Model file for the job. Use its own axes, mm. Face numbers are marked on the shaded views. A direction names the side the tool comes from. Round coordinates to 2 decimals unless told otherwise and drop trailing zeros. Order: outer loops, then holes, each group sorted by start corner. A loop starts at its lowest first (then second) coordinate and runs counter-clockwise, first axis right, second up. Notation, with made-up numbers: M 26,25.25 L 49,25.25 A25 ccw 49,64.25 Z; hole C 40.25,46.5 d5. An arc over 180 degrees is marked long. Return JSON: item names as keys, results as strings. Group by question number.
Item 1: Slice it at D-D on y = 83.5. Write the cut outline in (x, z), then the cut area to 3 significant figures.
Item 2: Slice it at B-B on y = 7. Write the cut outline in (x, z).
Item 3: Slice it at C-C on z = -30. Write the cut outline in (x, y), then the cut area to 3 significant figures.
Item 4: Pin check, flat tips, straight feed: pin 1 Ø3.5 at (x, y) = (89.9, 80) entering from +Z; pin 2 Ø5.5 at (x, y) = (89.9, 80) entering from -Z; pin 3 Ø1.5 at (x, z) = (34, -49) entering from +Y; pin 4 Ø5.5 at (x, z) = (70, -45) entering from -Y. Stop position of each tip, or through.
Item 5: Which spindle directions (+Z, -Z, +X, -X, +Y, -Y) get a long thin tool onto all of the face, cutting with end or side? Do the marked faces 1 and 2. Say none if no direction does.
Item 6: Probe line 1 along Z through (x, y) = (70, 6.5); line 2 along X through (y, z) = (80, -56); line 3 along X through (y, z) = (23.5, -30). List the from-to ranges inside material, lowest first.
Item 7: Pull direction X, two halves, no side cores. Call the marked faces 3, 4, 5 and 6: pulls with the +X half, pulls with the -X half, needs draft (parallel to the pull), parting line crosses it, or undercut.
Item 8: Slice it at A-A on x = 25. Write the cut outline in (y, z), then the cut area to 3 significant figures.
from build123d import *

# Parameters (mm, degrees)
SKETCH1_W                  = 100
SKETCH1_H                  = 100
BOSS_EXTRUDE1_DEPTH        = 100
SKETCH2_W                  = 60
SKETCH2_H                  = 100
CUT_EXTRUDE1_DEPTH         = 174.205080757
CUT_EXTRUDE2_DEPTH         = 157.212427483
CUT_EXTRUDE2_DEPTH_BACK    = 157.212427483
SKETCH3_R                  = 11
SKETCH4_W                  = 40
SKETCH4_H                  = 100
CUT_EXTRUDE3_DEPTH         = 174.205080757
BOSS_EXTRUDE2_START        = -10.65
SKETCH5_R                  = 11
SKETCH5_R_2                = 8
BOSS_EXTRUDE2_DEPTH        = 10.65
M5_TAPPED_HOLE1_AT_2_COUNT = 2
M5_TAPPED_HOLE1_AT_2_PITCH = 60
M5_TAPPED_HOLE2_D          = 4.2
M5_TAPPED_HOLE2_DEPTH      = 22
M5_TAPPED_HOLE2_TIP        = 1.2618073
M8_TAPPED_HOLE1_D          = 6.8
M8_TAPPED_HOLE1_DEPTH      = 24.25
M8_TAPPED_HOLE1_TIP        = 2.042926105
FILLET3_R                  = 10


with BuildPart() as part:
    # Sketch1 → Boss-Extrude1 (new body)
    with BuildSketch(Plane(origin=(0, 0, 0), x_dir=(1, 0, 0), z_dir=(0, 1, 0))):
        with Locations((50, 50)):
            Rectangle(SKETCH1_W, SKETCH1_H)
    extrude(amount=BOSS_EXTRUDE1_DEPTH)

    # Sketch2 → Cut-Extrude1 (cut, through all)
    with BuildSketch(Plane.XY):
        with Locations((30, 83.65)):
            Rectangle(SKETCH2_W, SKETCH2_H)
    extrude(amount=-CUT_EXTRUDE1_DEPTH, mode=Mode.SUBTRACT)

    # Sketch3 → Cut-Extrude2 (cut, two sides: drawn at the far end of the back side and taken through both)
    with BuildSketch(Plane(origin=(0, 33.65, 0), x_dir=(1, 0, 0), z_dir=(0, 1, 0)).offset(-CUT_EXTRUDE2_DEPTH_BACK)):
        with Locations(Location((25, 30, 0), (0, 0, 270))):
            Circle(SKETCH3_R)
    extrude(amount=CUT_EXTRUDE2_DEPTH + CUT_EXTRUDE2_DEPTH_BACK, mode=Mode.SUBTRACT)

    # Sketch4 → Cut-Extrude3 (cut, through all)
    with BuildSketch(Plane.ZY):
        with Locations((-80, 50)):
            Rectangle(SKETCH4_W, SKETCH4_H)
    extrude(amount=-CUT_EXTRUDE3_DEPTH, mode=Mode.SUBTRACT)

    # Sketch5 → Boss-Extrude2 (add)
    with BuildSketch(Plane.XZ.offset(BOSS_EXTRUDE2_START)):
        with Locations(Location((25, -30, 0), (0, 0, 270))):
            Circle(SKETCH5_R)
        with Locations(Location((25, -30, 0), (0, 0, 270))):
            Circle(SKETCH5_R_2, mode=Mode.SUBTRACT)
    extrude(amount=BOSS_EXTRUDE2_DEPTH)

    # Sketch11 → M5 Tapped Hole1 (revolve, cut)
    with BuildSketch(Plane(origin=(89.9, 80, 0), x_dir=(0, -1, 0), z_dir=(1, 0, 0))):
        Polygon((0, 0), (0, 16.2618073), (2.1, 15), (2.1, 0), align=None)
    m5_tapped_hole1 = revolve(axis=Axis((89.9, 80, 6.35), (0, 0, -1)), mode=Mode.SUBTRACT)

    # M5 Tapped Hole1 at 2: M5 Tapped Hole1 ×2
    with Locations(*[(0, -i * M5_TAPPED_HOLE1_AT_2_PITCH, 0) for i in range(1, M5_TAPPED_HOLE1_AT_2_COUNT)]):
        add(m5_tapped_hole1, mode=Mode.SUBTRACT)

    # Mirror1: M5 Tapped Hole1 across plane
    add(m5_tapped_hole1.mirror(Plane.XY.offset(-30)), mode=Mode.SUBTRACT)

    # Mirror1 copy 1 sketch → Mirror1 copy 1 (revolve, cut)
    with BuildSketch(Plane(origin=(89.9, 20, -60), x_dir=(0, -1, 0), z_dir=(1, 0, 0))):
        Polygon((0, 0), (0, -16.2618073), (2.1, -15), (2.1, 0), align=None)
    revolve(axis=Axis((89.9, 20, -66.35), (0, 0, -1)), mode=Mode.SUBTRACT)

    # M5 Tapped Hole2
    with Locations(Plane(origin=(0, 100, 0), x_dir=(1, 0, 0), z_dir=(0, 1, 0))):
        with Locations((70, 45), (70, 15)):
            Hole(M5_TAPPED_HOLE2_D / 2, depth=M5_TAPPED_HOLE2_DEPTH)
            with Locations((0, 0, -(M5_TAPPED_HOLE2_DEPTH + M5_TAPPED_HOLE2_TIP / 2))):  # 118° drill point
                Cone(0, M5_TAPPED_HOLE2_D / 2, M5_TAPPED_HOLE2_TIP, mode=Mode.SUBTRACT)

    # M8 Tapped Hole1
    with Locations(Plane(origin=(0, 0, 0), x_dir=(-1, 0, 0), z_dir=(0, -1, 0))):
        with Locations((-70, 15), (-70, 45)):
            Hole(M8_TAPPED_HOLE1_D / 2, depth=M8_TAPPED_HOLE1_DEPTH)
            with Locations((0, 0, -(M8_TAPPED_HOLE1_DEPTH + M8_TAPPED_HOLE1_TIP / 2))):  # 118° drill point
                Cone(0, M8_TAPPED_HOLE1_D / 2, M8_TAPPED_HOLE1_TIP, mode=Mode.SUBTRACT)

    # Fillet3
    fillet3_edges = [part.edges().sort_by_distance(p)[0] for p in [
        (0, 16.825, 0),
        (0, 16.825, -60),
    ]]
    fillet(fillet3_edges, radius=FILLET3_R)


solid = part.part
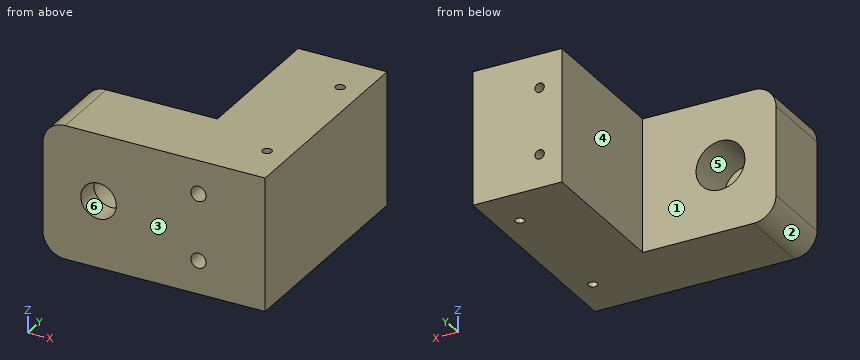
Output values:
{
 "1": {"outline": "M 60,-60 L 100,-60 L 100,0 L 60,0 Z; hole C 70,-45 d4.2; hole C 70,-15 d4.2", "area": "2,370 mm²"},
 "2": {"outline": "M 0,-50 A10 ccw 10,-60 L 100,-60 L 100,0 L 10,0 A10 ccw 0,-10 Z; hole C 25,-30 d16; hole C 70,-45 d6.8; hole C 70,-15 d6.8"},
 "3": {"outline": "M 0,0 L 17,0 L 17,10.65 L 14,10.65 L 14,33.65 L 0,33.65 Z; M 33,0 L 100,0 L 100,100 L 60,100 L 60,33.65 L 36,33.65 L 36,10.65 L 33,10.65 Z", "area": "5,340 mm²"},
 "4": {"pin 1": "z = -15.21", "pin 2": "z = -60", "pin 3": "y = 33.65", "pin 4": "y = 24.64"},
 "5": {"face 1": "+Z, -Z, -X, +Y", "face 2": "-Z, -X, +Y, -Y"},
 "6": {"line 1": "-60 to -48.4, -41.6 to -18.4, -11.6 to 0", "line 2": "60 to 87.8, 92 to 100", "line 3": "0 to 14, 36 to 100"},
 "7": {"face 3": "needs draft", "face 4": "pulls with the -X half", "face 5": "undercut", "face 6": "undercut"},
 "8": {"outline": "M 0,-60 L 33.65,-60 L 33.65,-41 L 10.65,-41 L 10.65,-38 L 0,-38 Z; M 0,-22 L 10.65,-22 L 10.65,-19 L 33.65,-19 L 33.65,0 L 0,0 Z", "area": "1,340 mm²"}
}
